from build123d import *

# Parameters (mm, degrees)
F0_R     = 12.7
F1_DEPTH = 76.2
F3_DEPTH = 50.8
F4_DEPTH = 12.7
F5_DEPTH = 25.4
F6_DEPTH = 12.7
F7_DEPTH = 25.4
F8_DEPTH = 76.2


with BuildPart() as f1:
    # F0 (on Right) → F1 (new body)
    with BuildSketch(Plane.YZ):
        with BuildLine():
            ThreePointArc((-12.7, 21.9970452561), (-12.7, -21.9970452561), (25.4, 0))
            ThreePointArc((25.4, 0), (12.7, 21.9970452561), (-12.7, 21.9970452561))
        make_face()
        Circle(F0_R, mode=Mode.SUBTRACT)
    extrude(amount=-F1_DEPTH)

    # F2 (on Front) → F3 (cut, symmetric)
    with BuildSketch(Plane.XZ):
        Polygon((-12.7, 9.525), (0, 9.525), (0, 25.4), (0, 50.8), (-76.2, 50.8), (-63.5, 38.1), (-50.8, 25.4), (-25.4, 25.4), (-25.4, 0), (-25.4, -9.525), (-12.7, -9.525), align=None)
    extrude(amount=F3_DEPTH, both=True, mode=Mode.SUBTRACT)

    # F2 (on Front) → F4 (join, symmetric)
    with BuildSketch(Plane.XZ):
        Polygon((-76.2, 38.1), (-76.2, 20.32), (-45.72, 20.32), (-50.8, 25.4), (-63.5, 38.1), align=None)
    extrude(amount=F4_DEPTH, both=True)

    # F2 (on Front) → F5 (join)
    with BuildSketch(Plane.XZ):
        Polygon((-76.2, 50.8), (-76.2, 38.1), (-63.5, 38.1), align=None)
        Polygon((-76.2, 38.1), (-76.2, 20.32), (-45.72, 20.32), (-50.8, 25.4), (-63.5, 38.1), align=None)
    extrude(amount=-F5_DEPTH)

    # F6 (cut): a face of the model
    f6_faces = [f1.faces().sort_by_distance(p)[0] for p in [
        (-71.9666666667, 0, 42.3333333333),
    ]]
    extrude(f6_faces, amount=-F6_DEPTH, mode=Mode.SUBTRACT)

    # F2 (on Front) → F7 (join, through all)
    with BuildSketch(Plane.XZ):
        Polygon((-76.2, 20.32), (-76.2, 0), (-25.4, 0), (-45.72, 20.32), align=None)
    extrude(amount=-F7_DEPTH)

    # F0 (on Right) → F8 (cut, through all)
    with BuildSketch(Plane.YZ):
        Circle(F0_R)
    extrude(amount=-F8_DEPTH, mode=Mode.SUBTRACT)


solid = f1.part
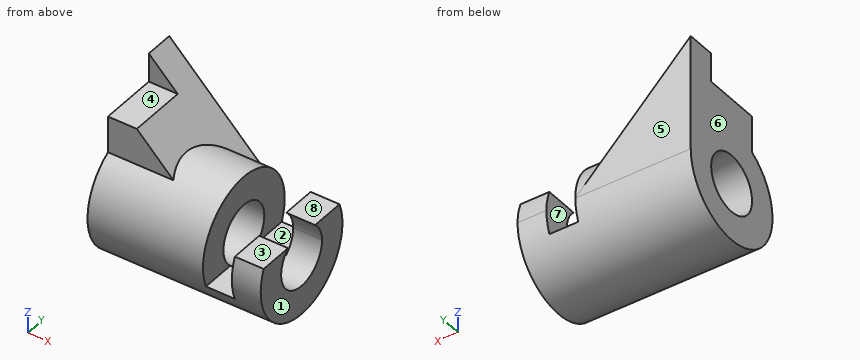
The model under review builds one solid part; all positions refer to its coordinate system, in mm. Face numbers are marked on the shaded views. A direction names the side the tool comes from. Give positions to 0.01 mm unless a question says otherwise; leave off trailing zeros. Order: outer loops, then holes, each group sorted by start corner. A loop starts at its lowest first (then second) coordinate and runs counter-clockwise, first axis right, second up. Notation, with made-up numbers: (-22.5, 76.5) -> (22.5, 76.5) arc R11 ccw to (22.5, 84.5) -> close; hole circle Ø4 at (-25, 89). An arc over 180 degrees is marked (long way). Write item = value, one per line. Start each with the question number.
(1) Take a section at C-C (z = -8). Write out the cut boundary in (x, y).
(2) Take a section at B-B (y = 5.5). Write out the cut boundary in (x, z).
(3) Tool access review of the marked faces 1, 2, 3, 4 and 5: name each direction out of +Z, -Z, +X, -X, +Y, -Y from which nothing blocks a thin tool from reaching the whole face with its end or side.
(4) Take a section at A-A (x = -54.5). Write out the cut boundary in (y, z).
(5) Take a section at D-D (y = -11). Write out the cut boundary in (x, z) (3 decimals), plus the area to 3 significant figures.
(6) Draft analysis for pull direction X (two halves, no side actions). For the marked faces 6, 7 and 8, state which applies: +X half, -X half, draft (parallel to the pull), parting line (faces both ways), or undercut.
(7) For L1, parallel to Z at x = -45, y = 0; L2, parallel to X at y = -14.5, z = 14; L3, parallel to Z at x = -25, y = 0, list the stretches that pass through material, from the lowest coordinate up. Write a range as from..to.
(8) For pin 1 Ø8 at (x, z) = (-59.5, 31) entering from -Y; pin 2 Ø6 at (x, z) = (-51.5, 15) entering from -Y; pin 3 Ø5 at (x, y) = (-37.5, 18) entering from +Z; pin 4 Ø15 at (y, z) = (0, 0) entering from -X, all flat-tipped, find the tip position at first contact; note any pin that passes through.
Returned:
q1.outline = (-76.2, -24.11) -> (-25.4, -24.11) -> (-25.4, -9.86) -> (-76.2, -9.86) -> close; (-76.2, 9.86) -> (-25.4, 9.86) -> (-25.4, 24.11) -> (-76.2, 24.11) -> close; (-12.7, -24.11) -> (0, -24.11) -> (0, -9.86) -> (-12.7, -9.86) -> close; (-12.7, 9.86) -> (0, 9.86) -> (0, 24.11) -> (-12.7, 24.11) -> close
q2.outline = (-76.2, -24.8) -> (0, -24.8) -> (0, -11.45) -> (-76.2, -11.45) -> close; (-76.2, 11.45) -> (-25.4, 11.45) -> (-25.4, 24.8) -> (-50.2, 24.8) -> (-63.5, 38.1) -> (-76.2, 38.1) -> close
q3.face_1 = +Z, -Z, +X, +Y, -Y
q3.face_2 = +Z, +Y, -Y
q3.face_3 = +Z, +X, +Y, -Y
q3.face_4 = +Z, +X, -X, -Y
q3.face_5 = +Z, -Z, +X, -X, +Y
q4.outline = (-12.7, 22) arc R25.4 ccw (long way) to (25.4, 0) -> (25.4, 29.1) -> (-12.7, 29.1) -> close; hole circle Ø25.4 at (0, 0)
q5.outline = (-76.2, -22.895) -> (0, -22.895) -> (0, -6.347) -> (-12.7, -6.347) -> (-12.7, -9.525) -> (-25.4, -9.525) -> (-25.4, -6.347) -> (-76.2, -6.347) -> close; (-76.2, 6.347) -> (-25.4, 6.347) -> (-25.4, 22.895) -> (-48.295, 22.895) -> (-63.5, 38.1) -> (-76.2, 38.1) -> close; (-12.7, 6.347) -> (0, 6.347) -> (0, 9.525) -> (-12.7, 9.525) -> close
q5.area = 2,410 mm²
q6.face_6 = -X half
q6.face_7 = undercut
q6.face_8 = draft
q7.L1 = -25.4..-12.7, 12.7..25.4
q7.L2 = -76.2..-25.4
q7.L3 = -25.4..-12.7
q8.pin_1 = -12.7
q8.pin_2 = -22.39
q8.pin_3 = 20.12
q8.pin_4 = through
